```python
from build123d import *

# Parameters (mm, degrees)
F0_W     = 279.4
F0_H     = 101.6
F1_DEPTH = 6.35
F2_DEPTH = 25.4
F3_T     = -6.35
F4_R     = 12.7


# Not quite as in the source:
# - a shell that OpenCascade refuses in one call is made with other operations: the cavity is built on its own and cut out


with BuildPart() as f1:
    # F0 (on Front) → F1 (new body)
    with BuildSketch(Plane.XZ):
        with Locations((0, -12.7)):
            Rectangle(F0_W, F0_H)
        Polygon((-139.7, 38.1), (139.7, 38.1), (139.7, 50.8), (0, 50.8), (-139.7, 50.8), align=None)
        Polygon((0, 50.8), (139.7, 50.8), (139.7, 63.5), (-139.7, 63.5), (-139.7, 50.8), align=None)
    extrude(amount=F1_DEPTH)

    # F0 (on Front) → F2 (join)
    with BuildSketch(Plane.XZ):
        Polygon((0, 50.8), (139.7, 50.8), (139.7, 63.5), (-139.7, 63.5), (-139.7, 50.8), align=None)
        Polygon((-139.7, 38.1), (139.7, 38.1), (139.7, 50.8), (0, 50.8), (-139.7, 50.8), align=None)
    extrude(amount=-F2_DEPTH)

    # F3: a shell. OpenCascade refuses it in one call, so the cavity is built on its own and cut out:
    # the body offset inwards by the wall thickness, plus a prism from it out through each open face.
    f3_core = offset(f1.part, amount=F3_T, kind=Kind.INTERSECTION, mode=Mode.PRIVATE)
    f3_exits = [f3_core.faces().sort_by_distance(p)[0] for p in [
        (0, 9.525, 44.45),
    ]]
    add(f3_core, mode=Mode.SUBTRACT)
    extrude(f3_exits, amount=-F3_T, mode=Mode.SUBTRACT)

    # F4
    f4_edges = [f1.edges().sort_by_distance(p)[0] for p in [
        (0, 25.4, 63.5),
    ]]
    fillet(f4_edges, radius=F4_R)


solid = f1.part
```
Build history of the part. All positions in model axes, mm. A direction names the side the tool comes from. Give positions to 0.01 mm unless a question says otherwise; leave off trailing zeros. Order: outer loops, then holes, each group sorted by start corner. A loop starts at its lowest first (then second) coordinate and runs counter-clockwise, first axis right, second up. Notation, with made-up numbers: M 27.25,-37 L 71.25,-37 A23 cw 71.25,-20 Z; hole C 12,89.25 d8. An arc over 180 degrees is marked long. Return JSON: item names as keys, results as strings.
Q1. Band-saw the part on B-B (y = 4.5). Give the cut face in (x, z).
Answer list:
{"outline": "M -139.7,38.1 L -133.35,38.1 L -133.35,57.15 L 133.35,57.15 L 133.35,38.1 L 139.7,38.1 L 139.7,63.5 L -139.7,63.5 Z"}
Q2. Wall check: probe 1 along X at (y, z) = (19, 45); probe 2 along Y at (x, z) = (-92, -3). Give the ranges that are in metal, low to high. Write a range as from..to.
Answer list:
{"probe 1": "x = -139.7..-133.35, 133.35..139.7", "probe 2": "y = -6.35..0"}
Q3. 3-axis set-ups, long thin cutter, end or side, ignore diameter. For faces 1 (the face through (-2, -6.35, 1)), 2 (the face through (2, 19.05, 48)), 3 (the face through (-0.7, 19.2, 38.1)): which of +Z, -Z, +X, -X, +Y, -Y reach the whole face in a straight line?
Answer list:
{"face 1": "+Z, -Z, +X, -X, -Y", "face 2": "-Z", "face 3": "-Z, +X, -X, +Y"}
Q4. Two-plate mould, pull along Y, no slides. Class faces 4 (the face through (-2, 25.4, 45)), 5 (the face through (-133.35, 9, 48)), 6 (the face through (2, 3, 63.5)), 7 (the face through (133.35, 9, 48)): pulls with the +Y half, pulls with the -Y half, needs draft (parallel to the pull), parting line crosses it, or undercut.
Answer list:
{"face 4": "pulls with the +Y half", "face 5": "undercut", "face 6": "needs draft", "face 7": "undercut"}
Q5. Flat gauge pins, fed straight in: pin 1 (1 mm diameter, centred on x = -37, z = 20, fed in from +Y); pin 2 (2 mm diameter, centred on x = 20, y = 20, fed in from -Z); pin 3 (2 mm diameter, centred on x = 46.5, y = 1.5, fed in from -Z). Where does each tip first touch, or does it go through?
Answer list:
{"pin 1": "stops at y = 0", "pin 2": "stops at z = 38.1", "pin 3": "stops at z = 57.15"}
Q6. Band-saw the part on A-A (x = 45.5). Give the cut face in (y, z), then the cut area to 3 significant figures.
Answer list:
{"outline": "M -6.35,-63.5 L 0,-63.5 L 0,57.15 L 19.05,57.15 L 19.05,38.1 L 25.4,38.1 L 25.4,50.8 A12.7 ccw 12.7,63.5 L -6.35,63.5 Z", "area": "1,050 mm^2"}
Q7. Band-saw the part on C-C (z = -52). Give the cut face in (x, y).
Answer list:
{"outline": "M -139.7,-6.35 L 139.7,-6.35 L 139.7,0 L -139.7,0 Z"}
